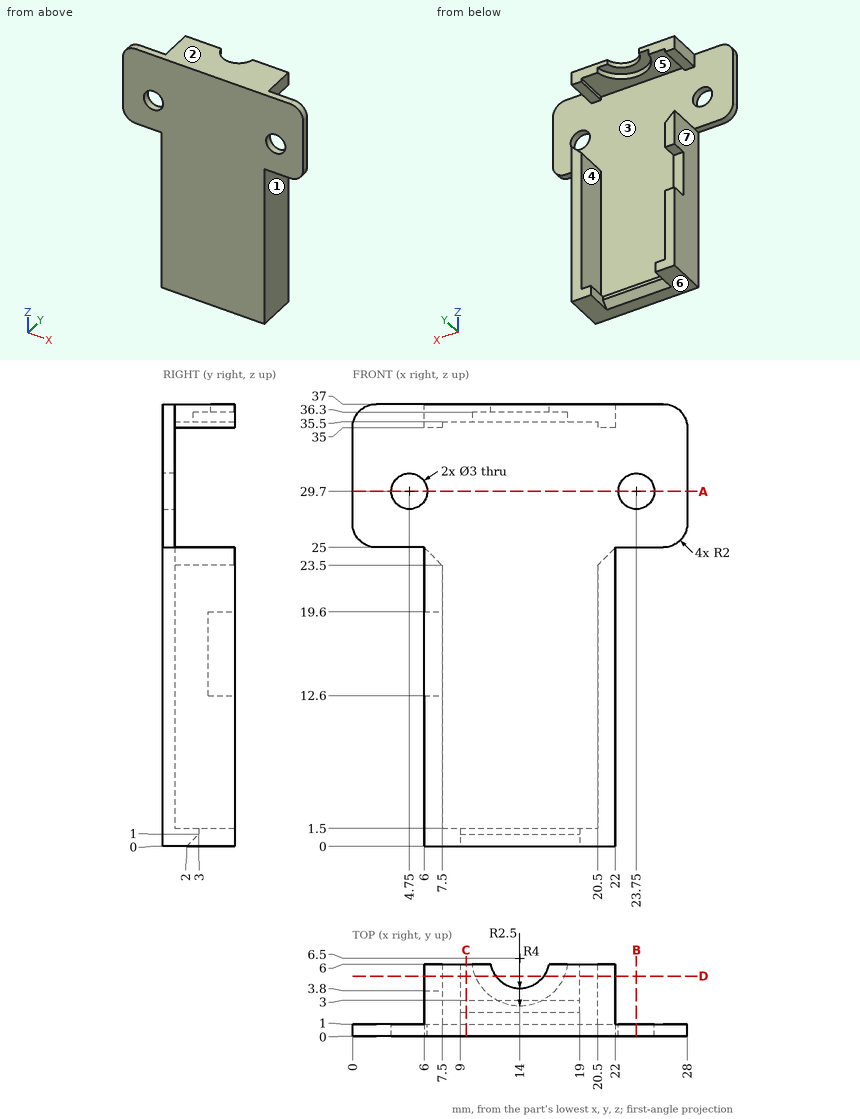
Design review of the part shown in the three views and the two pictorial views. Dimensions are in mm from the part's minimum x, y and z. A direction names the side the tool comes from. Give positions to 0.01 mm unless a question says otherwise; leave off trailing zeros. Loops run counter-clockwise (first coordinate to the right, second up) from the corner with the lowest first, then second, coordinate; pieces in that order, holes last. Notation, with made-up numbers: M 42,46.25 L 94,46.25 A13 cw 94,54.25 Z; hole C -24.75,82.25 d8. An arc over 180 degrees is marked long. Put each result on its own line as item: value. Start each with the question number.
(1) Add section A-A, the plane z = 29.7. Write out the cut boundary in (x, y).
(2) For pin 1 (2.5 mm diameter, centred on x = 23.75, z = 29.7, fed in from -Y); pin 2 (1.2 mm diameter, centred on x = 6.5, z = 15, fed in from +Y); pin 3 (1.5 mm diameter, centred on x = 14, z = 24.5, fed in from +Y); pin 4 (1.1 mm diameter, centred on x = 24, y = 0.5, fed in from -Z), all flat-tipped, find the tip position at first contact; note any pin that passes through.
(3) Machinability: for the marked faces 5, 6 and 7, which of the approach directions +Z, -Z, +X, -X, +Y, -Y give a long, thin tool a straight path to every point of the face, cutting with its end or side? Answer none if there is none.
(4) The part is to be moulded in two halves that separate along X. For the marked faces 1, 2, 3 and 4, say which applies: +X half, -X half, draft (parallel to the pull), parting line (faces both ways), or undercut.
(5) Add section B-B, the plane x = 23.75. Write out the cut boundary in (y, z), then the cut area to 3 significant figures.
(6) Add section D-D, the plane y = 5. Give the number of separate pieces and of enclosed holes in the cut face, then the cut area to 3 significant figures.
(7) Add section C-C, the plane x = 9.5. Write out the cut boundary in (y, z).
(8) Wall thickness on L1, parallel to X at y = 0.4, z = 29.7; L2, parallel to X at y = 5.75, z = 21; L3, parallel to Z at x = 8, y = 2.25: over which ranges is each line inside the solid? List them lowest first.
Result:
1. outline: M 0,0 L 3.25,0 L 3.25,1 L 0,1 Z; M 6.25,0 L 22.25,0 L 22.25,1 L 6.25,1 Z; M 25.25,0 L 28,0 L 28,1 L 25.25,1 Z
2. pin 1: passes through
2. pin 2: stops at y = 3.8
2. pin 3: stops at y = 1
2. pin 4: stops at z = 25
3. face 5: +Y
3. face 6: -Z, +X, -X, +Y, -Y
3. face 7: -Z, -X, +Y, -Y
4. face 1: +X half
4. face 2: draft
4. face 3: undercut
4. face 4: undercut
5. outline: M 0,25 L 1,25 L 1,28.2 L 0,28.2 Z; M 0,31.2 L 1,31.2 L 1,37 L 0,37 Z
5. area: 9.00 mm^2
6. separate pieces: 5
6. enclosed holes: 0
6. area: 83.5 mm^2
7. outline: M 0,0 L 2,0 L 3,1 L 3,1.5 L 1,1.5 L 1,35.5 L 6,35.5 L 6,37 L 0,37 Z
8. L1: x = 0 to 3.25, 6.25 to 22.25, 25.25 to 28
8. L2: x = 6 to 7.5, 20.5 to 22
8. L3: z = 0 to 1.5, 35.5 to 37
